Could you check a few things on this model? Use its own coordinates, in mm. Round coordinates to 2 decimals unless told otherwise and drop trailing zeros. Loops run counter-clockwise (first coordinate to the right, second up) from the corner with the lowest first, then second, coordinate; pieces in that order, holes last. Notation, with made-up numbers: (-36.5, 56) -> (22.5, 56) arc R20 cw to (22.5, 69) -> close; hole circle Ø10 at (-8, 7). An arc over 180 degrees is marked (long way). Write each question's results on one line, items separated by ' | '. Start each with the question number.
1) If I drill on probe 1 along Y at (x, z) = (0.4, 8); probe 2 along Z at (x, y) = (1.9, -6); probe 3 along Y at (x, z) = (0.35, 3.5), over which ranges is the centre line in solid material (lowest first)?
2) For P1, Ø8, axis at y = 2.5, z = -21, coming from the +X side; P2, Ø2, axis at y = 19, z = -13.5, coming from the -X side; P3, Ø2, axis at x = 3.5, y = -0.5, coming from the -Z side, each with a flat end and sliding along its axis, tell me the tip position at first contact or that it passes through.
3) Imagine slicing it at A-A, the plane z = 0. List the corners of the cut face in (x, y) for me.
4) We'd pull the mould along Y, two halves only. Please class faces 1 (the flat face through (0, 18, -18)), 2 (the cylindrical face through (4.872, 25.896, -8.155)), 3 (the cylindrical face through (3.038, 23.846, 7.509)): pulls with the +Y half, pulls with the -Y half, needs draft (parallel to the pull), parting line crosses it, or undercut.
5) Imagine slicing it at C-C, the plane x = 4.55. List the corners of the cut face in (y, z) for me, plus the area to 3 significant figures.
Autodesk Inventor part; units mm, degrees
ref_plane "ir_XY" through (0, 0, 0) normal (0, 0, 1) x (1, 0, 0)
ref_plane "ir_YZ" through (0, 0, 0) normal (1, 0, 0) x (0, 1, 0)
ref_plane "ir_ZX" through (0, 0, 0) normal (0, 1, 0) x (0, 0, 1)
sketch "Sketch_10" plane through (0, 0, 0) normal (0, 0, 1) x (1, 0, 0)
  line L0 (50, 0) -> (-50, 0)
  line L1 (0, 27.09) -> (0, 25.3)
  arc A0 (0, 25.3) -> (0.3, 25) centre (0.3, 25.3) ccw
  line L2 (0.3, 25) -> (5.7, 25)
  arc A1 (5.7, 25) -> (6, 25.3) centre (5.7, 25.3) ccw
  line L3 (6, 25.3) -> (6, 27.09)
  arc A2 (6, 27.09) -> (5.94, 27.15) centre (5.94, 27.09) ccw
  line L4 (5.94, 27.15) -> (3.8335, 27.15)
  arc A3 (2.1665, 27.15) -> (3.8335, 27.15) centre (3, 28) ccw
  line L5 (2.1665, 27.15) -> (0.06, 27.15)
  arc A4 (0.06, 27.15) -> (0, 27.09) centre (0.06, 27.09) ccw
revolve "Revolution1" add sketch "Sketch_10" angle 360 about axis through (50, 0, 0) along (1, 0, 0)
ref_plane "ir_XY" through (0, 0, 0) normal (0, 0, 1) x (1, 0, 0)
ref_plane "ir_YZ" through (0, 0, 0) normal (1, 0, 0) x (0, 1, 0)
ref_plane "ir_ZX" through (0, 0, 0) normal (0, 1, 0) x (0, 0, 1)
properties part number "SKF_W 61710_ir"
Checked values:
1) probe 1: -25.94 to -23.69, 23.69 to 25.94 | probe 2: -26.48 to -24.27, 24.27 to 26.48 | probe 3: -26.92 to -24.75, 24.75 to 26.92
2) P1: x = 5.96 | P2: through | P3: z = -27.15
3) outline: (0, -27.09) arc R0.06 ccw to (0.06, -27.15) -> (2.17, -27.15) arc R1.19 cw to (3.83, -27.15) -> (5.94, -27.15) arc R0.06 ccw to (6, -27.09) -> (6, -25.3) arc R0.3 ccw to (5.7, -25) -> (0.3, -25) arc R0.3 ccw to (0, -25.3) -> close; (0, 25.3) arc R0.3 ccw to (0.3, 25) -> (5.7, 25) arc R0.3 ccw to (6, 25.3) -> (6, 27.09) arc R0.06 ccw to (5.94, 27.15) -> (3.83, 27.15) arc R1.19 cw to (2.17, 27.15) -> (0.06, 27.15) arc R0.06 ccw to (0, 27.09) -> close
4) face 1: needs draft | face 2: parting line crosses it | face 3: undercut
5) outline: circle Ø54.3 at (0, 0); hole circle Ø50 at (0, 0) | area: 352 mm^2
